from build123d import *

# Parameters (mm, degrees)
BOSS_EXTRUDE1_DEPTH                          = 25
SKETCH2_W                                    = 13.175144841
SKETCH2_H                                    = 18.76358654
SKETCH2_W_2                                  = 10
SKETCH2_W_3                                  = 19.622994234
CUT_EXTRUDE1_DEPTH                           = 11
CUT_EXTRUDE1_DEPTH_BACK                      = 3
FILLET1_R                                    = 20
CSK_FOR_M4_COUNTERSUNK_FLAT_HEAD_SCR_2_COUNT = 2
CSK_FOR_M4_COUNTERSUNK_FLAT_HEAD_SCR_2_PITCH = 20.373860658
CSK_FOR_M4_COUNTERSUNK_FLAT_HEAD_SCR_3_COUNT = 2
CSK_FOR_M4_COUNTERSUNK_FLAT_HEAD_SCR_3_PITCH = 20.021215351


with BuildPart() as part:
    # Sketch1 → Boss-Extrude1 (new body, symmetric)
    with BuildSketch(Plane.XY):
        with BuildLine():
            Line((0, 0), (0, 50))
            ThreePointArc((0, 50), (11.186683916, 53.016340491), (3.032769985, 44.785065097))
            Line((3.032769985, 44.785065097), (4.021846657, 46.523376732))
            ThreePointArc((4.021846657, 46.523376732), (9.457789277, 52.01089366), (2, 50))
            Line((2, 50), (2, 0))
            Line((2, 0), (0, 0))
        make_face()
    extrude(amount=BOSS_EXTRUDE1_DEPTH, both=True)

    # Sketch2 → Cut-Extrude1 (cut, two sides)
    with BuildSketch(Plane(origin=(2, 0, 0), x_dir=(0, 0, -1), z_dir=(1, 0, 0))) as cut_extrude1_sk:
        with Locations((-21.587572421, 51.660780085)):
            Rectangle(SKETCH2_W, SKETCH2_H)
        with Locations((0, 51.660780085)):
            Rectangle(SKETCH2_W_2, SKETCH2_H)
        with Locations((24.811497117, 51.660780085)):
            Rectangle(SKETCH2_W_3, SKETCH2_H)
    extrude(amount=CUT_EXTRUDE1_DEPTH, mode=Mode.SUBTRACT)
    extrude(cut_extrude1_sk.sketch, amount=-CUT_EXTRUDE1_DEPTH_BACK, mode=Mode.SUBTRACT)

    # Fillet1
    fillet1_edges = [part.edges().sort_by_distance(p)[0] for p in [
        (1, 0, 25),
        (1, 0, -25),
    ]]
    fillet(fillet1_edges, radius=FILLET1_R)

    # Sketch4 → CSK for M4 Countersunk Flat Head Screw1 (revolve, cut)
    with BuildSketch(Plane(origin=(2, 11.587467643, 0), x_dir=(0, 0, -1), z_dir=(0, 1, 0))):
        Polygon((0, 0), (0, 2), (2.25, 2), (2.25, 2.45), (4.7, 0), align=None)
    csk_for_m4_countersunk_flat_head_screw1 = revolve(axis=Axis((8.35, 11.587467643, 0), (-1, 0, 0)), mode=Mode.SUBTRACT)

    # CSK for M4 Countersunk Flat Head Scr 2: CSK for M4 Countersunk Flat Head Screw1 ×2
    with Locations(*[Vector(0, 0.807519759, 0.58984052) * (i * CSK_FOR_M4_COUNTERSUNK_FLAT_HEAD_SCR_2_PITCH) for i in range(1, CSK_FOR_M4_COUNTERSUNK_FLAT_HEAD_SCR_2_COUNT)]):
        add(csk_for_m4_countersunk_flat_head_screw1, mode=Mode.SUBTRACT)

    # CSK for M4 Countersunk Flat Head Scr 3: CSK for M4 Countersunk Flat Head Screw1 ×2
    with Locations(*[Vector(0, 0.77172393, -0.635957683) * (i * CSK_FOR_M4_COUNTERSUNK_FLAT_HEAD_SCR_3_PITCH) for i in range(1, CSK_FOR_M4_COUNTERSUNK_FLAT_HEAD_SCR_3_COUNT)]):
        add(csk_for_m4_countersunk_flat_head_screw1, mode=Mode.SUBTRACT)


solid = part.part
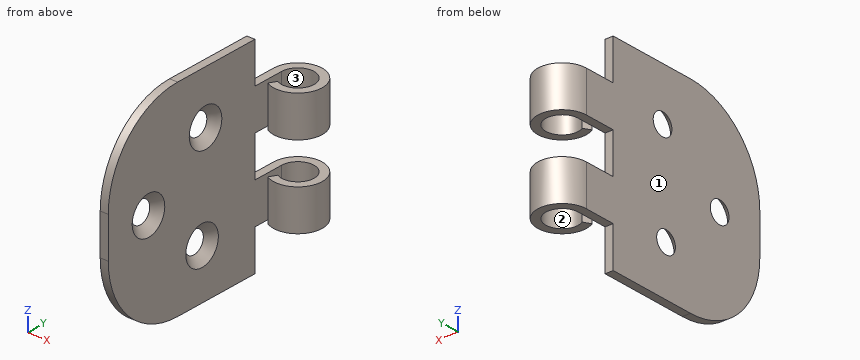
Work out the finished part from the listing and answer in its coordinate system (mm). Face numbers are marked on the shaded views. Round coordinates to 2 decimals unless told otherwise and drop trailing zeros. Order: outer loops, then holes, each group sorted by start corner. A loop starts at its lowest first (then second) coordinate and runs counter-clockwise, first axis right, second up. Notation, with made-up numbers: M -8,-5.5 L 2,-5.5 A19 ccw 2,11.5 Z; hole C 28.25,33 d1. An arc over 180 degrees is marked long. Put each result on its own line as item: value. Start each with the question number.
Q1. For a pull along X with two mould halves and no side action, classify the marked faces 1, 2 and 3 as pulls with the +X half, pulls with the -X half, needs draft (parallel to the pull), parting line crosses it, or undercut.
Q2. Section A-A, the plane y = 48 is taken. Write down the section's boundary in (x, z), and give its area (3 significant figures).
Q3. Section D-D, the plane x = 1 is taken. Write down the section's boundary in (y, z).
Q4. Straight lines are drawn through the part: L1, parallel to Y at x = 6, z = -10.75; L2, parallel to X at y = 50, z = 9.5; L3, parallel to Z at x = 8, y = 46. For each, find the intervals that lie inside material, in ascending order. Write a range as [from, to].
Q5. Section B-B, the plane x = 8 is taken. Write down the section's boundary in (y, z), and give its area (3 significant figures).
Q6. Flat-ended cylindrical pins translate along their axes: pin 1 (2 mm diameter, centred on x = 1, z = 22, fed in from +Y); pin 2 (1 mm diameter, centred on x = 2, z = -10.5, fed in from +Y); pin 3 (4 mm diameter, centred on x = 10.5, z = -10.5, fed in from +Y); pin 4 (6 mm diameter, centred on x = 7, y = 34.5, fed in from +Z). Find the tip coordinate at first contact, or state that the pin passes through.
Q7. Section C-C, the plane z = 0 is taken. Write down the section's boundary in (x, y), and give its area (3 significant figures).
Findings below:
1. face 1: pulls with the -X half
1. face 2: undercut
1. face 3: undercut
2. outline: M 0,-15 L 2,-15 L 2,-5 L 0,-5 Z; M 0,5 L 2,5 L 2,15 L 0,15 Z; M 9.46,-15 L 11.66,-15 L 11.66,-5 L 9.46,-5 Z; M 9.46,5 L 11.66,5 L 11.66,15 L 9.46,15 Z
2. area: 83.9 mm^2
3. outline: M 0,-5 A20 ccw 20,-25 L 42.28,-25 L 42.28,-15 L 53.32,-15 L 53.32,-5 L 42.28,-5 L 42.28,5 L 53.32,5 L 53.32,15 L 42.28,15 L 42.28,25 L 20,25 A20 ccw 0,5 Z; hole C 11.59,0 d7.4; hole C 27.04,-12.73 d7.4; hole C 28.04,12.02 d7.4
4. L1: y = [44, 46], [54, 56]
4. L2: x = [0, 2], [10, 12]
4. L3: z = [-15, -5], [5, 15]
5. outline: M 44.34,-15 L 46.54,-15 L 46.54,-5 L 44.34,-5 Z; M 44.34,5 L 46.54,5 L 46.54,15 L 44.34,15 Z; M 53.46,-15 L 55.66,-15 L 55.66,-5 L 53.46,-5 Z; M 53.46,5 L 55.66,5 L 55.66,15 L 53.46,15 Z
5. area: 87.7 mm^2
6. pin 1: stops at y = 42.28
6. pin 2: stops at y = 54.87
6. pin 3: stops at y = 55.45
6. pin 4: passes through
7. outline: M 0,0 L 2,0 L 2,6.89 L 0,8.89 Z; M 0,14.29 L 2,16.29 L 2,42.28 L 0,42.28 Z
7. area: 69.8 mm^2
